Autodesk Inventor part; units mm, degrees
ref_plane "YZ Plane" through (0, 0, 0) normal (1, 0, 0) x (0, 1, 0)
ref_plane "XZ Plane" through (0, 0, 0) normal (0, 1, 0) x (-1, 0, 0)
ref_plane "XY Plane" through (0, 0, 0) normal (0, 0, 1) x (1, 0, 0)
sketch "Sketch1" plane through (0, 0, 0) normal (0, 0, 1) x (1, 0, 0)
  line L0 (57.5, 0) -> (28.75, -49.7965)
  line L1 (28.75, -49.7965) -> (-28.75, -49.7965)
  line L2 (-28.75, -49.7965) -> (-57.5, 0)
  line L3 (-57.5, 0) -> (-28.75, 49.7965)
  line L4 (-28.75, 49.7965) -> (28.75, 49.7965)
  line L5 (28.75, 49.7965) -> (57.5, 0)
  point P0 (0, 0)
  point P1 (0, 0)
  dimension "d0" = 115
extrude "Extrusion1" add sketch "Sketch1" along normal blind 139.4929
sketch "Sketch2" plane through (-28.75, -49.7965, 0) normal (0, -1, 0) x (1, 0, 0)
  line L0 (-28.75, 89.6965) -> (0, 139.4929)
  line L1 (0, 139.4929) -> (57.5, 139.4929)
  line L2 (57.5, 139.4929) -> (86.25, 89.6965)
  line L3 (86.25, 89.6965) -> (57.5, 39.9)
  line L4 (57.5, 39.9) -> (0, 39.9)
  line L5 (0, 39.9) -> (-28.75, 89.6965)
  line L6 (0, 139.4929) -> (57.5, 139.4929)
  point P0 (28.75, 0)
  point P1 (28.75, 89.6965)
  point P2 (28.75, 139.4929)
  dimension "d3" = 115
extrude "Extrusion2" add sketch "Sketch2" against normal blind 307.5
sketch "Sketch3" plane through (0, 0, 139.4929) normal (0, 0, 1) x (1, 0, 0)
  line L0 (-28.75, 49.7965) -> (-28.75, 257.7035)
  line L1 (-28.75, 100.2035) -> (-100, 100.2035)
  line L2 (-100, 100.2035) -> (-100, 257.7035)
  line L3 (-57.5, 257.7035) -> (-28.75, 257.7035)
  line L4 (-100, 257.7035) -> (-28.75, 257.7035)
  line L5 (-80, 100.2035) -> (-100, 120.2035)
  point P0 (0, 0)
  dimension "d6" = 71.25
  dimension "d7" = 157.5
  dimension "d8" = 28.2843
  dimension "d9" = 45
extrude "Extrusion3" add sketch "Sketch3" against normal blind 99.5929 contours L1 L5 L2 L4 L3 L0
sketch "Sketch4" plane through (-100, 120.2035, 139.4929) normal (-1, 0, 0) x (0, 0, 1)
  line L0 (-99.5929, 94.375) -> (-74.6947, 137.5)
  line L1 (-74.6947, 137.5) -> (-24.8982, 137.5)
  line L2 (-24.8982, 137.5) -> (0, 94.375)
  line L3 (0, 94.375) -> (-24.8982, 51.25)
  line L4 (-24.8982, 51.25) -> (-74.6947, 51.25)
  line L5 (-74.6947, 51.25) -> (-99.5929, 94.375)
  line L6 (0, 137.5) -> (-99.5929, 137.5)
  line L7 (0, 137.5) -> (0, 0)
  line L8 (-99.5929, 0) -> (-99.5929, 137.5)
  point P0 (-139.4929, -120.2035)
  point P1 (-49.7965, 94.375)
  point P2 (-49.7965, 137.5)
extrude "Extrusion4" add sketch "Sketch4" against normal blind 180 contours L0 L1 L2 L3 L4 L5
sketch "Sketch6" plane through (80, 120.2035, 139.4929) normal (1, 0, 0) x (0, 0, -1)
  line L0 (0, 94.375) -> (24.8982, 137.5)
  line L1 (0, 137.5) -> (24.8982, 137.5)
  line L2 (0, 94.375) -> (0, 137.5)
  line L3 (74.6947, 137.5) -> (99.5929, 94.375)
  line L4 (99.5929, 94.375) -> (99.5929, 137.5)
  line L5 (74.6947, 137.5) -> (99.5929, 137.5)
  line L6 (49.7965, -120.2035) -> (99.5929, -170)
  line L7 (49.7965, -170) -> (49.7965, -120.2035)
  line L8 (99.5929, -170) -> (49.7965, -170)
  line L9 (0, -170) -> (49.7965, -120.2035)
  line L10 (49.7965, -170) -> (0, -170)
  line L11 (49.7965, -170) -> (49.7965, -120.2035)
  line L12 (0, -170) -> (49.7965, -120.2035)
  line L13 (49.7965, -120.2035) -> (0, -120.2035)
  line L14 (0, -170) -> (0, -120.2035)
  line L15 (49.7965, -120.2035) -> (0, -70.4071)
  line L16 (0, -120.2035) -> (0, -70.4071)
  line L17 (49.7965, -120.2035) -> (0, -120.2035)
  point P0 (139.4929, -120.2035)
extrude "Extrusion5" cut sketch "Sketch6" against normal through all
sketch "Sketch7" plane through (0, 0, 0) normal (0, 0, -1) x (-1, 0, 0)
  circle A0 centre (0, 0) radius 25
  dimension "d16" = 50
extrude "Extrusion6" cut sketch "Sketch7" against normal blind 5
sketch "Sketch8" plane through (80, 120.2035, 139.4929) normal (1, 0, 0) x (0, 0, -1)
  line L0 (74.6947, 51.25) -> (99.5929, 94.375)
  line L1 (99.5929, 94.375) -> (74.6947, 137.5)
  line L2 (74.6947, 137.5) -> (24.8982, 137.5)
  line L3 (24.8982, 137.5) -> (0, 94.375)
  line L4 (0, 94.375) -> (24.8982, 51.25)
  line L5 (24.8982, 51.25) -> (74.6947, 51.25)
  circle A0 centre (49.7965, 94.375) radius 25
  point P0 (139.4929, -120.2035)
  point P1 (49.7965, 137.5)
  dimension "d19" = 50
extrude "Extrusion7" add sketch "Sketch8" along normal blind 5 contours A0
sketch "Sketch9" plane through (0, 0, 139.4929) normal (0, 0, 1) x (1, 0, 0)
  line L0 (-57.5, 0) -> (-57.5, 100.2035)
  line L1 (-57.5, 60.2035) -> (57.5, 60.2035)
  line L2 (57.5, 60.2035) -> (57.5, -49.7965)
  line L3 (57.5, -49.7965) -> (-57.5, -49.7965)
  line L4 (-57.5, -49.7965) -> (-57.5, 60.2035)
  line L5 (57.5, 0) -> (57.5, 171.4535)
  line L6 (28.75, -49.7965) -> (-28.75, -49.7965)
  line L7 (-80, 100.2035) -> (-28.75, 100.2035)
  point P0 (0, 0)
  point P1 (0, -49.7965)
  dimension "d22" = 40
extrude "Extrusion8" cut sketch "Sketch9" against normal through all
sketch "Sketch10" plane through (-28.75, 60.2035, 139.4929) normal (0, -1, 0) x (1, 0, 0)
  line L0 (57.5, 0) -> (86.25, -49.7965)
  line L1 (0, 0) -> (57.5, 0)
  line L2 (-28.75, -49.7965) -> (0, 0)
  line L3 (0, -99.5929) -> (-28.75, -49.7965)
  line L4 (57.5, -99.5929) -> (0, -99.5929)
  line L5 (86.25, -49.7965) -> (57.5, -99.5929)
  circle A0 centre (28.75, -49.7965) radius 25
  point P0 (28.75, -139.4929)
  point P1 (28.75, 0)
  dimension "d25" = 50
extrude "Extrusion9" cut sketch "Sketch10" against normal blind 5 contours A0
properties part number "link_a0" material "ABS Plastic"
Part model, mm, in its own coordinate system. A direction names the side the tool comes from. Round coordinates to 2 decimals unless told otherwise and drop trailing zeros. Loops run counter-clockwise (first coordinate to the right, second up) from the corner with the lowest first, then second, coordinate; pieces in that order, holes last.
1. Flat gauge pins, fed straight in: pin 1 (2 mm diameter, centred on x = 41.5, z = 123.5, fed in from -Y); pin 2 (10 mm diameter, centred on y = 97, z = 106, fed in from -X); pin 3 (25 mm diameter, centred on x = 7.5, z = 89.5, fed in from -Y). Where does each tip first touch, or does it go through?
Solutions:
pin 1: stops at y = 185.15
pin 2: stops at x = -81.8
pin 3: stops at y = 65.2
2. Drill centre lines: line 1 along Z through (x, y) = (0, 63.85); line 2 along Y through (x, z) = (75, 93.5); line 3 along Y through (x, z) = (22.5, 83.5). Where is each one in solid material? Low to high.
Solutions:
line 1: z = 39.9 to 64.7, 114.7 to 139.49
line 2: y = 171.45 to 257.7
line 3: y = 65.2 to 257.7
3. 3-axis set-ups, long thin cutter, end or side, ignore diameter. For faces 5 (the face through (0, 65.204, 90)), 6 (the face through (42.924, 119.158, 114.943)), 7 (the face through (-42.924, 79.923, 64.45)): which of +Z, -Z, +X, -X, +Y, -Y reach the whole face in a straight line?
Solutions:
face 5: -Y
face 6: +Z, +X, -Y
face 7: -Z, -X, -Y
4. Slice it at C-C (y = 150). Give the cut face in (x, z), and give its area (3 significant figures).
Solutions:
outline: (-100, 39.9) - (28.75, 39.9) - (57.5, 89.7) - (28.75, 139.49) - (-100, 139.49) - close
area: 14,300 mm2
5. Slice it at B-B (z = 120.5). Give the cut face in (x, y), and give its area (3 significant figures).
Solutions:
outline: (-100, 120.2) - (-80, 100.2) - (-39.72, 100.2) - (-39.72, 60.2) - (39.72, 60.2) - (39.72, 181.68) - (80, 181.68) - (80, 247.48) - (-100, 247.48) - close
area: 26,200 mm2
6. Slice it at A-A (x = 0). Give the cut face in (y, z), and give its area (3 significant figures).
Solutions:
outline: (60.2, 39.9) - (214.58, 39.9) - (257.7, 64.8) - (257.7, 114.59) - (214.58, 139.49) - (60.2, 139.49) - (60.2, 114.7) - (65.2, 114.7) - (65.2, 64.7) - (60.2, 64.7) - close
area: 18,300 mm2
7. Slice it at D-D (z = 80). Give the cut face in (x, y), and give its area (3 significant figures).
Solutions:
outline: (-100, 120.2) - (-80, 100.2) - (-51.9, 100.2) - (-51.9, 60.2) - (-23.04, 60.2) - (-23.04, 65.2) - (23.04, 65.2) - (23.04, 60.2) - (51.9, 60.2) - (51.9, 171.45) - (80, 171.45) - (80, 191.54) - (85, 191.54) - (85, 237.62) - (80, 237.62) - (80, 257.7) - (-100, 257.7) - close
area: 30,300 mm2
8. Two-plate mould, pull along Z, no slides. Class faces 1 (the face through (11.5, 62.7, 67.5)), 2 (the face through (-11.26, 235.839, 52.175)), 3 (the face through (85, 215, 90)), 4 (the face through (-37, 156, 139.493)): pulls with the +Z half, pulls with the -Z half, needs draft (parallel to the pull), parting line crosses it, or undercut.
Solutions:
face 1: undercut
face 2: pulls with the -Z half
face 3: needs draft
face 4: pulls with the +Z half
